```python
from build123d import *

# Parameters (mm, degrees)
CROQUIS1_W              = 17
CROQUIS1_H              = 15
SALIENTE_EXTRUIR1_DEPTH = 32
CROQUIS1_3_W            = 11.5
CROQUIS1_3_H            = 15
SALIENTE_EXTRUIR2_DEPTH = 10
CROQUIS2_R              = 2.75
CORTAR_EXTRUIR1_DEPTH   = 20
CROQUIS3_R              = 2.5
CORTAR_EXTRUIR2_DEPTH   = 20
CROQUIS4_R              = 1.5
CORTAR_EXTRUIR3_DEPTH   = 20


with BuildPart() as part:
    # Croquis1 → Saliente-Extruir1 (new body)
    with BuildSketch(Plane(origin=(0, 0, 0), x_dir=(1, 0, 0), z_dir=(0, 1, 0))):
        Rectangle(CROQUIS1_W, CROQUIS1_H)
    extrude(amount=SALIENTE_EXTRUIR1_DEPTH)

    # Croquis1_3 → Saliente-Extruir2 (add)
    with BuildSketch(Plane(origin=(0, 0, 0), x_dir=(1, 0, 0), z_dir=(0, 1, 0))):
        with Locations((-14.25, 0)):
            Rectangle(CROQUIS1_3_W, CROQUIS1_3_H)
        with Locations((14.25, 0)):
            Rectangle(CROQUIS1_3_W, CROQUIS1_3_H)
    extrude(amount=SALIENTE_EXTRUIR2_DEPTH)

    # Croquis2 → Cortar-Extruir1 (cut)
    with BuildSketch(Plane(origin=(0, 0, -7.5), x_dir=(-1, 0, 0), z_dir=(0, 0, -1))):
        with Locations((0, 25)):
            Circle(CROQUIS2_R)
        with BuildLine():
            Line((0.5, 32), (-0.5, 32))
            Line((-0.5, 32), (-0.5, 27.704163457))
            ThreePointArc((-0.5, 27.704163457), (0, 27.75), (0.5, 27.704163457))
            Line((0.5, 27.704163457), (0.5, 32))
        make_face()
    extrude(amount=-CORTAR_EXTRUIR1_DEPTH, mode=Mode.SUBTRACT)

    # Croquis3 → Cortar-Extruir2 (cut)
    with BuildSketch(Plane(origin=(0, 10, 0), x_dir=(1, 0, 0), z_dir=(0, 1, 0))):
        with Locations((14.25, 0)):
            Circle(CROQUIS3_R)
        with Locations((-14.25, 0)):
            Circle(CROQUIS3_R)
    extrude(amount=-CORTAR_EXTRUIR2_DEPTH, mode=Mode.SUBTRACT)

    # Croquis4 → Cortar-Extruir3 (cut)
    with BuildSketch(Plane.ZY.offset(8.5)):
        with Locations((0, 24.943618043)):
            Circle(CROQUIS4_R)
    extrude(amount=-CORTAR_EXTRUIR3_DEPTH, mode=Mode.SUBTRACT)


solid = part.part
```
The model under review builds one solid part; all positions refer to its coordinate system, in mm. A direction names the side the tool comes from. Give positions to 0.01 mm unless a question says otherwise; leave off trailing zeros. Write each loop counter-clockwise with the first axis right and the second up, starting at its lowest first coordinate (ties: lowest second). Pieces come first, ordered by that corner, then holes. Notation, with made-up numbers: M -38.5,3.25 L 6.5,3.25 A22 ccw 6.5,13.25 Z; hole C 7.5,79 d7. An arc over 180 degrees is marked long. Write each question's results on one line, items separated by ' | '. Start each with the question number.
1. We need section D-D (z = -3.5). Write out the cut boundary in (x, y).
2. We need section A-A (y = 28.5). Write out the cut boundary in (x, z), and give its area (3 significant figures).
3. We need section B-B (x = 14.25). Write out the cut boundary in (y, z).
4. Mouldability with a two-part tool opening along X and no side actions: class faces 4 (the flat face through (11.6, 10, -0.1)), 5 (the cylindrical face through (11.752, 5.07, -0.11)), 6 (the cylindrical face through (-16.748, 5.07, -0.11)), 7 (the flat face through (8.5, 21, 0)) as released by +X, released by -X, zero draft, split by the parting line, or undercut.
5. We need section C-C (y = 2). Write out the cut boundary in (x, z), and give its area (3 significant figures).
6. Insertion check: pin 1 Ø3.5 at (y, z) = (30.5, -1) entering from +X; pin 2 Ø1.5 at (y, z) = (15.5, 3.5) entering from -X; pin 3 Ø1 at (x, z) = (-9.5, 1) entering from +Y. Each pin has a flat end and moves straight along its axis. Give the tip position at first contact, or say it passes through.
7. For faces 1 (the flat face through (0.5, 30, 0)), 2 (the flat face through (0, 9, 7.5)), 3 (the flat face through (-8.5, 21, 0)), list the 3-axis set-ups (+Z, -Z, +X, -X, +Y, -Y) from which the entire face can be reached by the end or side of a thin tool; tool diameter is ignored.
8. For probe 1 along X at (y, z) = (7.75, 0); probe 2 along X at (y, z) = (30.5, -7); probe 3 along X at (y, z) = (9.5, -0.75), list the stretches that pass through material, from the lowest coordinate up. Write a range as [from, to].
Results found:
1) outline: M -20,0 L 20,0 L 20,10 L 8.5,10 L 8.5,32 L 0.5,32 L 0.5,27.7 A2.75 cw long -0.5,27.7 L -0.5,32 L -8.5,32 L -8.5,10 L -20,10 Z
2) outline: M -8.5,-7.5 L -0.5,-7.5 L -0.5,7.5 L -8.5,7.5 Z; M 0.5,-7.5 L 8.5,-7.5 L 8.5,7.5 L 0.5,7.5 Z | area: 240 mm^2
3) outline: M 0,-7.5 L 10,-7.5 L 10,-2.5 L 0,-2.5 Z; M 0,2.5 L 10,2.5 L 10,7.5 L 0,7.5 Z
4) face 4: zero draft | face 5: undercut | face 6: undercut | face 7: released by +X
5) outline: M -20,-7.5 L 20,-7.5 L 20,7.5 L -20,7.5 Z; hole C -14.25,0 d5; hole C 14.25,0 d5 | area: 561 mm^2
6) pin 1: stops at x = 8.5 | pin 2: stops at x = -8.5 | pin 3: stops at y = 10
7) face 1: +Z, -Z, +Y | face 2: +Z, +X, -X, +Y, -Y | face 3: +Z, -Z, -X, +Y
8) probe 1: x = [-20, -16.75], [-11.75, 11.75], [16.75, 20] | probe 2: x = [-8.5, -0.5], [0.5, 8.5] | probe 3: x = [-20, -16.63], [-11.87, 11.87], [16.63, 20]
